Source: CAD feature listing. Evaluate the final solid. Frame: model axes, mm. Give positions to 0.01 mm unless a question says otherwise; leave off trailing zeros. Loops run counter-clockwise (first coordinate to the right, second up) from the corner with the lowest first, then second, coordinate; pieces in that order, holes last.
from build123d import *

# Parameters (mm, degrees)
SKETCH1_R           = 14.2875
BOSS_EXTRUDE1_DEPTH = 7.62
SKETCH2_R           = 14.2875
SKETCH2_R_2         = 2.5527
CUT_EXTRUDE1_DEPTH  = 8.62
SKETCH5_W           = 25.4
SKETCH5_H           = 25.4
SKETCH5_R           = 3.175
BOSS_EXTRUDE3_DEPTH = 7.62
BOSS_EXTRUDE4_DEPTH = 7.62
SKETCH7_R           = 3.175
CUT_EXTRUDE2_DEPTH  = 8.62
CUT_EXTRUDE3_DEPTH  = 7.62


with BuildPart() as part:
    # Sketch1 → Boss-Extrude1 (new body)
    with BuildSketch(Plane(origin=(0, 0, 0), x_dir=(1, 0, 0), z_dir=(0, 1, 0))):
        Polygon((-76.2, 14.749121283), (-14.331263069, -20.970810639), (25.4, -20.970810639), (25.4, 13.954189361), (-50.8, 62.374121283), (-152.4, 62.374121283), (-152.4, 14.749121283), align=None)
        Circle(SKETCH1_R, mode=Mode.SUBTRACT)
    extrude(amount=BOSS_EXTRUDE1_DEPTH)

    # Sketch2 → Cut-Extrude1 (cut, through all)
    with BuildSketch(Plane(origin=(0, 7.62, 0), x_dir=(1, 0, 0), z_dir=(0, 1, 0))):
        with Locations((-78.335649741, 38.561621283)):
            Circle(SKETCH2_R)
        with Locations((-103.087949741, 38.561621283)):
            Circle(SKETCH2_R_2)
        with Locations((-53.583349741, 38.561621283)):
            Circle(SKETCH2_R_2)
    extrude(amount=-CUT_EXTRUDE1_DEPTH, mode=Mode.SUBTRACT)

    # Sketch5 → Boss-Extrude3 (add)
    with BuildSketch(Plane(origin=(0, 7.62, 0), x_dir=(1, 0, 0), z_dir=(0, 1, 0))):
        with Locations((38.1, -8.270810639)):
            Rectangle(SKETCH5_W, SKETCH5_H)
        with Locations((38.1, -1.920810639)):
            Circle(SKETCH5_R, mode=Mode.SUBTRACT)
    extrude(amount=-BOSS_EXTRUDE3_DEPTH)

    # Sketch6 → Boss-Extrude4 (add)
    with BuildSketch(Plane(origin=(0, 7.62, 0), x_dir=(1, 0, 0), z_dir=(0, 1, 0))):
        Polygon((-152.4, -23.350878717), (-127, -23.350878717), (-114.3, 14.749121283), (-152.4, 14.749121283), (-152.4, 62.374121283), (-158.75, 62.374121283), (-158.75, -23.350878717), align=None)
    extrude(amount=-BOSS_EXTRUDE4_DEPTH)

    # Sketch7 → Cut-Extrude2 (cut, through all)
    with BuildSketch(Plane(origin=(0, 7.62, 0), x_dir=(1, 0, 0), z_dir=(0, 1, 0))):
        with Locations((-139.7, 21.480121283)):
            Circle(SKETCH7_R)
        with Locations((-139.7, -3.919878717)):
            Circle(SKETCH7_R)
    extrude(amount=-CUT_EXTRUDE2_DEPTH, mode=Mode.SUBTRACT)

    # Sketch10 → Cut-Extrude3 (cut)
    with BuildSketch(Plane(origin=(0, 7.62, 0), x_dir=(1, 0, 0), z_dir=(0, 1, 0))):
        Polygon((-76.2, 14.749121283), (-69.85, 14.749121283), (-7.981263069, -20.970810639), (-14.331263069, -20.970810639), align=None)
    extrude(amount=-CUT_EXTRUDE3_DEPTH, mode=Mode.SUBTRACT)


solid = part.part
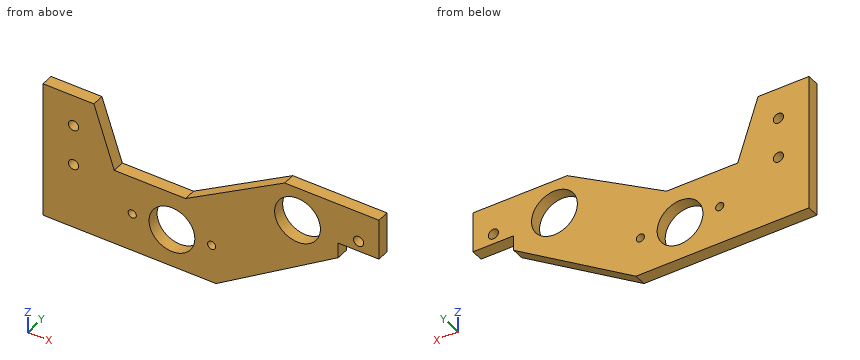
1) Cut plane D-D (y = 5). State how many separate pieces and enclosed holes the cut face has, and give its area (3 significant figures).
Checks:
separate pieces: 1
enclosed holes: 7
area: 9,900 mm2
2) Cut plane A-A (x = -139.7). Return loops of the section in (y, z), and give its area (3 significant figures).
Checks:
outline: (0, -62.37) - (7.62, -62.37) - (7.62, -24.66) - (0, -24.66) - close; (0, -18.31) - (7.62, -18.31) - (7.62, 0.74) - (0, 0.74) - close; (0, 7.09) - (7.62, 7.09) - (7.62, 23.35) - (0, 23.35) - close
area: 556 mm2
3) Ray query, probe 1 along Z at (x, y) = (-139.7, 4.25); probe 2 along X at (y, z) = (3.5, 0); probe 3 along X at (y, z) = (6.25, 3). Return the intervals inside material, ascending.
Checks:
probe 1: z = -62.37 to -24.66, -18.31 to 0.74, 7.09 to 23.35
probe 2: x = -158.75 to -119.22, -44.3 to -14.29, 14.29 to 35.57, 40.63 to 50.8
probe 3: x = -158.75 to -142.74, -136.66 to -120.22, -39.11 to -13.97, 13.97 to 35.11, 41.09 to 50.8
4) Cut plane B-B (z = -28.5). Return loops of the section in (x, y), and give its area (3 significant figures).
Checks:
outline: (-158.75, 0) - (-88.48, 0) - (-88.48, 7.62) - (-158.75, 7.62) - close; (-68.19, 0) - (2.51, 0) - (2.51, 7.62) - (-68.19, 7.62) - close
area: 1,070 mm2
5) Cut plane C-C (x = 38.1). Return loops of the section in (y, z).
Checks:
outline: (0, -4.43) - (7.62, -4.43) - (7.62, -1.25) - (0, -1.25) - close; (0, 5.1) - (7.62, 5.1) - (7.62, 20.97) - (0, 20.97) - close
6) Contact query for flat-ended pins moving along their axis: P1, Ø4, axis at x = 33.5, y = 2, coming from the -Z side; P2, Ø3, axis at x = 15.5, y = 3.5, coming from the +Z side; P3, Ø5, axis at x = -139.7, z = 3.92, coming from the -Y side; P4, Ø3, axis at y = 2.5, z = -50.5, coming from the +X side. Output: stop coordinate, or through.
Checks:
P1: stops at z = -4.43
P2: stops at z = 20.97
P3: passes through
P4: stops at x = -29.75
